```python
from build123d import *

# Parameters (mm, degrees)
SKETCH_1_W      = 12
SKETCH_1_H      = 38
SKETCH_1_R      = 2.5
EXTRUDE_1_DEPTH = 1
EXTRUDE_2_DEPTH = 7.8
EXTRUDE_START   = -30.2
EXTRUDE_3_DEPTH = 7.8


with BuildPart() as part:
    # 草图1 → 凸台-拉伸1 (new body)
    with BuildSketch(Plane.XY):
        with Locations((6, 19)):
            Rectangle(SKETCH_1_W, SKETCH_1_H)
        with Locations((6, 31.5)):
            Circle(SKETCH_1_R, mode=Mode.SUBTRACT)
        with Locations((6, 6.5)):
            Circle(SKETCH_1_R, mode=Mode.SUBTRACT)
    extrude(amount=EXTRUDE_1_DEPTH)

    # 草图2 → 凸台-拉伸2 (add)
    with BuildSketch(Plane(origin=(0, 38, 0), x_dir=(1, 0, 0), z_dir=(0, 1, 0))):
        with BuildLine():
            Line((12, 0), (17, 0))
            ThreePointArc((17, 0), (20.535533906, -8.535533906), (12, -5))
            Line((12, -5), (13, -5))
            ThreePointArc((13, -5), (19.828427125, -7.828427125), (17, -1))
            Line((17, -1), (12, -1))
            Line((12, -1), (12, 0))
        make_face()
    extrude(amount=-EXTRUDE_2_DEPTH)

    # 草图2<2> → 凸台-拉伸3 (add)
    with BuildSketch(Plane(origin=(0, 38, 0), x_dir=(1, 0, 0), z_dir=(0, 1, 0)).offset(EXTRUDE_START)):
        with BuildLine():
            Line((12, 0), (17, 0))
            ThreePointArc((17, 0), (20.535533906, -8.535533906), (12, -5))
            Line((12, -5), (13, -5))
            ThreePointArc((13, -5), (19.828427125, -7.828427125), (17, -1))
            Line((17, -1), (12, -1))
            Line((12, -1), (12, 0))
        make_face()
    extrude(amount=-EXTRUDE_3_DEPTH)


solid = part.part
```
Verification items for the finished model (mm, model axes). A direction names the side the tool comes from. Coordinates: 2 decimals unless noted, no trailing zeros. Loops run counter-clockwise (first coordinate to the right, second up) from the corner with the lowest first, then second, coordinate; pieces in that order, holes last. Notation, with made-up numbers: (79, 29.5) - (90, 29.5) arc R26 ccw to (90, 59.5) - close; hole circle Ø7 at (-22, 26.5). An arc over 180 degrees is marked (long way). Put each result on its own line as item: value.
Item 1: Section check D-D (y = 21.5). Enter the section's corners in (x, z).
Conclusion:
outline: (0, 0) - (12, 0) - (12, 1) - (0, 1) - close
Item 2: Gauge pin test, flat ends, axial feed: pin 1 Ø2 at (x, z) = (13.5, 3.5) entering from +Y; pin 2 Ø8 at (x, y) = (9, 4) entering from +Z; pin 3 Ø1 at (x, y) = (5.5, 20) entering from +Z. Record the tip position at first contact, or that the pin passes through.
Conclusion:
pin 1: passes through
pin 2: stops at z = 8
pin 3: stops at z = 1
Item 3: Scan lines: line 1 along Y through (x, z) = (6, 0.4); line 2 along Z through (x, y) = (17, 2.75); line 3 along X through (y, z) = (3.5, 7.25). Record each from-to range of solid material in increasing order.
Conclusion:
line 1: y = 0 to 4, 9 to 29, 34 to 38
line 2: z = 0 to 1, 9 to 10
line 3: x = 12.53 to 13.69, 20.31 to 21.47
Item 4: Set-up check for faces 1 (the face through (12.7, 38, 5.3)), 2 (the face through (12, 18.8, 0.5)), 3 (the face through (12.5, 4, 5)): record each of +Z, -Z, +X, -X, +Y, -Y from which the full face is reachable in a straight line by a thin tool's end or side.
Conclusion:
face 1: +Z, -Z, +X, -X, +Y
face 2: +Z, -Z, +X
face 3: -X, +Y, -Y
Item 5: Section check C-C (z = 8). Enter the section's corners in (x, y).
Conclusion:
outline: (13, 0) - (14.35, 0) - (14.35, 7.8) - (13, 7.8) - close; (13, 30.2) - (14.35, 30.2) - (14.35, 38) - (13, 38) - close; (19.65, 0) - (21, 0) - (21, 7.8) - (19.65, 7.8) - close; (19.65, 30.2) - (21, 30.2) - (21, 38) - (19.65, 38) - close
Item 6: Section check A-A (x = 6). Enter the section's corners in (y, z), then the cut area to 3 significant figures.
Conclusion:
outline: (0, 0) - (4, 0) - (4, 1) - (0, 1) - close; (9, 0) - (29, 0) - (29, 1) - (9, 1) - close; (34, 0) - (38, 0) - (38, 1) - (34, 1) - close
area: 28.0 mm2
Item 7: Draft check along Y on faces 4 (the face through (8.385, 7.251, 0.493)), 5 (the face through (12.7, 0, 5.3)), 6 (the face through (19.734, 34.155, 7.92)). Enter one of: pulls with the +Y half, pulls with the -Y half, needs draft (parallel to the pull), parting line crosses it, or undercut.
Conclusion:
face 4: undercut
face 5: pulls with the -Y half
face 6: needs draft
Item 8: Section check B-B (y = 32). Enter the section's corners in (x, z).
Conclusion:
outline: (0, 0) - (3.55, 0) - (3.55, 1) - (0, 1) - close; (8.45, 0) - (17, 0) arc R5 ccw (long way) to (12, 5) - (13, 5) arc R4 cw (long way) to (17, 1) - (8.45, 1) - close
